Can you work these out from the model? Positions are in its coordinate system, mm. A direction names the side the tool comes from. Round coordinates to 2 decimals unless told otherwise and drop trailing zeros. Order: outer loops, then holes, each group sorted by start corner. A loop starts at its lowest first (then second) coordinate and runs counter-clockwise, first axis right, second up. Notation, with made-up numbers: (63, -36.5) - (103, -36.5) arc R31 cw to (103, -3.5) - close; hole circle Ø8 at (-39.5, 88.5). An arc over 180 degrees is marked (long way). Write item = value, one per line.
Autodesk Inventor part; units mm, degrees
ref_plane "YZ Plane" through (0, 0, 0) normal (1, 0, 0) x (0, 1, 0)
ref_plane "XZ Plane" through (0, 0, 0) normal (0, 1, 0) x (-1, 0, 0)
ref_plane "XY Plane" through (0, 0, 0) normal (0, 0, 1) x (1, 0, 0)
sketch "Sketch1" plane through (0, 0, 0) normal (1, 0, 0) x (0, 1, 0)
  line L0 (11.9118, 21.1765) -> (-8.0882, 21.1765)
  line L1 (-8.0882, 21.1765) -> (-8.0882, -23.8235)
  line L2 (-8.0882, -23.8235) -> (11.9118, -23.8235)
  line L3 (11.9118, -23.8235) -> (11.9118, 21.1765)
  point P0 (0, 0)
  dimension "d0" = 45
  dimension "d1" = 20
extrude "Extrusion1" add sketch "Sketch1" along normal blind 2
sketch "Sketch2" plane through (2, 0, 0) normal (1, 0, 0) x (0, 0, -1)
  circle A0 centre (-9.1765, 1.9118) radius 8.5
  circle A1 centre (11.8235, 1.9118) radius 8.5
  line L0 (23.8235, 11.9118) -> (-21.1765, 11.9118)
  line L1 (-21.1765, 11.9118) -> (-21.1765, -8.0882)
  line L2 (23.8235, -8.0882) -> (23.8235, 11.9118)
  point P0 (0, 0)
  dimension "d4" = 17
  dimension "d5" = 10
  dimension "d6" = 10
  dimension "d7" = 12
  dimension "d8" = 12
extrude "Extrusion2" add sketch "Sketch2" along normal blind 13
sketch "Sketch3" plane through (15, 1.9118, 9.1765) normal (1, 0, 0) x (0, 0, -1)
  circle A0 centre (0, 0) radius 6.5
  circle A1 centre (21, 0) radius 6.5
  circle A2 centre (21, 0) radius 8.5
  circle A3 centre (0, 0) radius 8.5
  point P0 (9.1765, -1.9118)
  dimension "d11" = 13
extrude "Extrusion3" cut sketch "Sketch3" against normal blind 2 contours A0 | A1
equation "\"d6\" = d5"
equation "\"d8\" = d7"
properties part number "Sonar"
(1) If we section it at A-A (z = 9.5): Write out the boundary of the cut face in (x, y), plus the area to 3 significant figures.
Computed:
outline = (0, -8.09) - (2, -8.09) - (2, -6.58) - (15, -6.58) - (15, -4.58) - (13, -4.58) - (13, 8.4) - (15, 8.4) - (15, 10.41) - (2, 10.41) - (2, 11.91) - (0, 11.91) - close
area = 235 mm^2
(2) If we section it at C-C (y = 0.75): Write out the boundary of the cut face in (x, z).
Computed:
outline = (0, -23.82) - (2, -23.82) - (2, -20.24) - (15, -20.24) - (15, -18.22) - (13, -18.22) - (13, -5.43) - (15, -5.43) - (15, -3.4) - (2, -3.4) - (2, 0.76) - (15, 0.76) - (15, 2.78) - (13, 2.78) - (13, 15.57) - (15, 15.57) - (15, 17.6) - (2, 17.6) - (2, 21.18) - (0, 21.18) - close
(3) On a 3-axis mill with a long thin cutter (end or side, diameter ignored), from which of +Z, -Z, +X, -X, +Y, -Y can I reach the whole of each face in a straight line? I mean faces 5 (the face through (15, -3.1, -16.2)), 6 (the face through (14.014, -2.043, -6.665)). Say none if no direction works.
Computed:
face_5 = +Z, -Z, +X, +Y, -Y
face_6 = +X
(4) If we section it at D-D (x = 11.25): Write out the boundary of the cut face in (y, z).
Computed:
outline = circle Ø17 at (1.91, -11.82); circle Ø17 at (1.91, 9.18)
(5) Thinking about a two-plate mould opening in Z: for faces 1 (the face through (2, 2, -1)), 2 (the face through (13, 2, -12)), 3 (the face through (1, 11.912, -2)), 4 (the face through (1, 2, 21.176)), which applies, +Z half, -Z half, draft (parallel to the pull), parting line (faces both ways), or undercut?
Computed:
face_1 = undercut
face_2 = undercut
face_3 = draft
face_4 = +Z half
(6) If I drill on line 1 (Y direction, x = 10.75, z = -12); line 2 (X direction, y = -5.5, z = -2.5); line 3 (X direction, y = 1, z = -12.5), over which ranges is the centre line in solid material (lowest first)? Write a range as from..to.
Computed:
line_1 = -6.59..10.41
line_2 = 0..2
line_3 = 0..13
(7) If we section it at B-B (x = 14.25): Write out the boundary of the cut face in (y, z), plus the area to 3 significant figures.
Computed:
outline = circle Ø17 at (1.91, -11.82); circle Ø17 at (1.91, 9.18); hole circle Ø13 at (1.91, -11.82); hole circle Ø13 at (1.91, 9.18)
area = 188 mm^2
(8) Will these pins go through, and if not, where does the flat tip stop? P1, Ø10, axis at y = 5, z = -9.5, coming from the -X side; P2, Ø2, axis at x = 4, z = -11.5, coming from the -Y side; P3, Ø6.5, axis at y = 4, z = -11, coming from the +X side; P4, Ø2, axis at x = 13, y = 0.5, coming from the +Z side.
Computed:
P1 = 0
P2 = -6.59
P3 = 13
P4 = 17.67
